Autodesk Inventor part; units mm, degrees
ref_plane "YZ Plane" through (0, 0, 0) normal (1, 0, 0) x (0, 1, 0)
ref_plane "XZ Plane" through (0, 0, 0) normal (0, 1, 0) x (-1, 0, 0)
ref_plane "XY Plane" through (0, 0, 0) normal (0, 0, 1) x (1, 0, 0)
sketch "草圖1" plane through (0, 0, 0) normal (0, 0, 1) x (1, 0, 0)
  circle A0 centre (0, 0) radius 47
  circle A1 centre (40.0673, -8.6957) radius 2.5 construction
  circle A2 centre (-8.6957, -40.0673) radius 2.5 construction
  circle A3 centre (-40.0673, 8.6957) radius 2.5 construction
  circle A4 centre (8.6957, 40.0673) radius 2.5 construction
  circle A5 centre (0, 0) radius 41 construction
  circle A6 centre (41, 0) radius 2.5
  circle A7 centre (0, 41) radius 2.5
  circle A8 centre (-41, 0) radius 2.5
  circle A9 centre (0, -41) radius 2.5
  point P0 (0, 0)
  dimension "d11" = 5
  dimension "d14" = 360
extrude "擠出1" add sketch "草圖1" along normal blind 6
sketch "草圖3" plane through (0, 0, 6) normal (0, 0, 1) x (1, 0, 0)
  circle A0 centre (0, 0) radius 4
  dimension "d4" = 8
extrude "擠出3" cut sketch "草圖3" against normal through all
sketch "草圖6" plane through (0, 0, 6) normal (0, 0, 1) x (1, 0, 0)
  circle A0 centre (9.4848, 3.1685) radius 2.5 construction
  circle A1 centre (-9.4848, -3.1685) radius 2.5 construction
  circle A2 centre (3.1685, -9.4848) radius 2.5 construction
  circle A3 centre (-3.1685, 9.4848) radius 2.5 construction
  circle A4 centre (0, 0) radius 21
  circle A5 centre (0, 0) radius 4
  circle A6 centre (0, 0) radius 10 construction
  circle A7 centre (10, 0) radius 2.5
  circle A8 centre (0, 10) radius 2.5
  circle A9 centre (-10, 0) radius 2.5
  circle A10 centre (0, -10) radius 2.5
  point P0 (0, 0)
  dimension "d16" = 5
  dimension "d19" = 360
extrude "擠出5" cut sketch "草圖6" against normal through all contours A7 | A8 | A9 | A10
sketch "草圖10" plane through (0, 0, 6) normal (0, 0, 1) x (1, 0, 0)
  circle A0 centre (-19.8414, 19.8414) radius 1.5
  line L0 (-21.9203, 26.163) -> (-26.163, 21.9203)
  line L1 (-26.163, 21.9203) -> (-25.4983, 21.2556)
  line L2 (-25.4983, 21.2556) -> (-21.2556, 25.4983)
  line L3 (-21.2556, 25.4983) -> (-21.9203, 26.163)
  line L4 (0, 0) -> (-33.234, 33.234) construction
  line L5 (0, 0) -> (18.5986, 0) construction
  circle A1 centre (0, 0) radius 47
  point P0 (-23.377, 23.377)
  dimension "d30" = 3
  dimension "d31" = 0.94
  dimension "d35" = 5
  dimension "d38" = 135
  dimension "d39" = 6
  dimension "d40" = 34
extrude "擠出7" cut sketch "草圖10" against normal through all contours A0 | L3 L2 L1 L0
sketch "草圖11" plane through (0, 0, 6) normal (0, 0, 1) x (1, 0, 0)
  circle A0 centre (-19.8414, 19.8414) radius 1.5
  line L0 (-21.2556, 25.4983) -> (-25.4983, 21.2556)
  line L1 (-25.4983, 21.2556) -> (-26.163, 21.9203)
  line L2 (-26.163, 21.9203) -> (-21.9203, 26.163)
  line L3 (-21.9203, 26.163) -> (-21.2556, 25.4983)
  circle A1 centre (-10, 0) radius 2.5
  circle A2 centre (0, 10) radius 2.5
  circle A3 centre (0, -10) radius 2.5
  circle A4 centre (10, 0) radius 2.5
  circle A5 centre (0, 0) radius 4
  circle A6 centre (0, 0) radius 47
  circle A7 centre (0, -41) radius 2.5
  circle A8 centre (-41, 0) radius 2.5
  circle A9 centre (0, 41) radius 2.5
  circle A10 centre (41, 0) radius 2.5
chamfer "倒角1" distance 2.5 angle 45 4 edges at (-2.5, -41, 0) (38.5, 0, 0) (-43.5, 0, 0) (-2.5, 41, 0)
properties part number "base gear base plate"
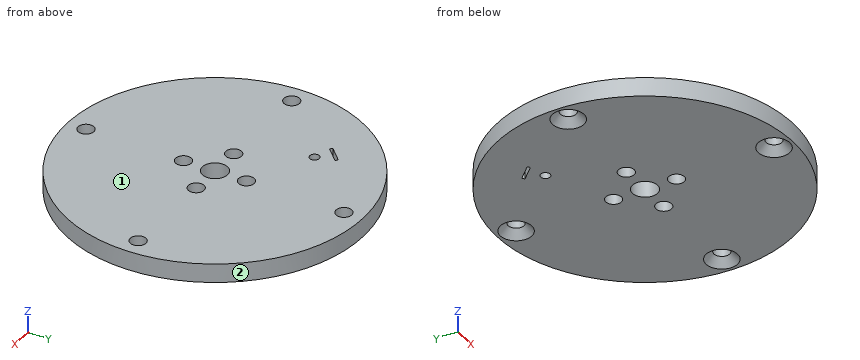
Geometry: final body of the model. Coordinates: model frame, mm. Face numbers are marked on the shaded views. Round coordinates to 2 decimals unless told otherwise and drop trailing zeros. Order: outer loops, then holes, each group sorted by start corner. A loop starts at its lowest first (then second) coordinate and runs counter-clockwise, first axis right, second up. Notation, with made-up numbers: (12.5, 65.5) - (61.5, 65.5) arc R21 ccw to (61.5, 76.5) - close; hole circle Ø1 at (24.5, 67.5). An arc over 180 degrees is marked (long way). Write item = value, one per line. Start each with the question number.
Q1. Cut plane C-C on z = 4. Give the number of separate pieces and of enclosed holes in the cut face, and give its area (3 significant figures).
Q2. Pin query (flat end, axial travel): pin 1 (1.5 mm diameter, centred on y = 22, z = 2, fed in from -X); pin 2 (4 mm diameter, centred on x = 41, y = 0, fed in from -Z); pin 3 (6 mm diameter, centred on x = -41, y = 0, fed in from -Z); pin 4 (8 mm diameter, centred on x = 0, y = -41, fed in from -Z). Return the tip coordinate at first contact, or that it passes through.
Q3. Cut plane A-A on y = 0. Return the cut outline in (x, z), and give its area (4 significant figures).
Q4. Cut plane D-D on y = -10. Return the cut outline in (x, z), and give its area (3 significant figures).
Q5. Ray query, line 1 (Y direction, x = 0, z = 3.3); line 2 (Y direction, x = 10, z = 4.4); line 3 (X direction, y = 21, z = 1.95). Return the intervals inside material, ascending. Write a range as from..to.
Q6. Pull-direction query (Y, two-part tool) for the marked faces 1 and 2; classes: +Y half, -Y half, draft (parallel to the pull), parting line (faces both ways), or undercut.
Q7. Cut plane B-B on x = -19.5. Return the cut outline in (y, z).
Outcome:
q1.separate_pieces = 1
q1.enclosed_holes = 11
q1.area = 6,720 mm^2
q2.pin_1 = -41.92
q2.pin_2 = through
q2.pin_3 = 2
q2.pin_4 = 1
q3.outline = (-47, 0) - (-46, 0) - (-43.5, 2.5) - (-43.5, 6) - (-47, 6) - close; (-38.5, 2.5) - (-36, 0) - (-12.5, 0) - (-12.5, 6) - (-38.5, 6) - close; (-7.5, 0) - (-4, 0) - (-4, 6) - (-7.5, 6) - close; (4, 0) - (7.5, 0) - (7.5, 6) - (4, 6) - close; (12.5, 0) - (36, 0) - (38.5, 2.5) - (38.5, 6) - (12.5, 6) - close; (43.5, 2.5) - (46, 0) - (47, 0) - (47, 6) - (43.5, 6) - close
q3.area = 383.5 mm^2
q4.outline = (-45.92, 0) - (-2.5, 0) - (-2.5, 6) - (-45.92, 6) - close; (2.5, 0) - (45.92, 0) - (45.92, 6) - (2.5, 6) - close
q4.area = 521 mm^2
q5.line_1 = -47..-43.5, -38.5..-12.5, -7.5..-4, 4..7.5, 12.5..38.5, 43.5..47
q5.line_2 = -45.92..-2.5, 2.5..45.92
q5.line_3 = -42.05..-20.79, -18.89..42.05
q6.face_1 = draft
q6.face_2 = parting line
q7.outline = (-42.76, 0) - (18.38, 0) - (18.38, 6) - (-42.76, 6) - close; (21.3, 0) - (42.76, 0) - (42.76, 6) - (21.3, 6) - close
